Model file for the job. Use its own axes, mm. A direction names the side the tool comes from. Round coordinates to 2 decimals unless told otherwise and drop trailing zeros. Loops run counter-clockwise (first coordinate to the right, second up) from the corner with the lowest first, then second, coordinate; pieces in that order, holes last. Notation, with made-up numbers: (-33.5, 44.25) -> (-15.5, 44.25) arc R14 cw to (-15.5, 63.25) -> close; hole circle Ø3 at (10.25, 50). An arc over 180 degrees is marked (long way). Use a Markdown table: item, result. Add a question column.
```python
from build123d import *

# Parameters (mm, degrees)
F3_DEPTH = 9
F5_DEPTH = 47


with BuildPart() as f1:
    # F0 (on Front) → F1 (revolve)
    with BuildSketch(Plane.XZ):
        Polygon((-5.6564239193, 9.5), (-5.6564239193, 7.5), (19.3435760807, 7.5), (19.3435760807, 9.5), (31.3435760807, 9.5), (31.3435760807, 11.5), (-15.6564239193, 11.5), (-15.6564239193, 9.5), align=None)
    revolve(axis=Axis((2.8128489057, 0, 0), (1, 0, 0)))

    # F2 (on face) → F3 (join)
    with BuildSketch(Plane.YZ.offset(19.3435760807)):
        with BuildLine():
            Line((0, 7.5), (0, 9.5))
            ThreePointArc((0, 9.5), (-1.2098512295, 9.4226461253), (-2.4, 9.191844211))
            Line((-2.4, 9.191844211), (-2.4, 7.5))
            Line((-2.4, 7.5), (0, 7.5))
        make_face()
        with BuildLine():
            ThreePointArc((2.4, 9.191844211), (1.2098512295, 9.4226461253), (0, 9.5))
            Line((0, 9.5), (0, 7.5))
            Line((0, 7.5), (2.4, 7.5))
            Line((2.4, 7.5), (2.4, 9.191844211))
        make_face()
    extrude(amount=F3_DEPTH)

    # F4 (on face) → F5 (join, through all)
    with BuildSketch(Plane.YZ.offset(31.3435760807)):
        with BuildLine():
            Line((-15, -11.5), (0, -11.5))
            ThreePointArc((0, -11.5), (-4.1533119315, -10.7238052948), (-7.7459666924, -8.5))
            Line((-7.7459666924, -8.5), (-15, -8.5))
            Line((-15, -8.5), (-15, -11.5))
        make_face()
        with BuildLine():
            ThreePointArc((7.7459666924, -8.5), (4.1533119315, -10.7238052948), (0, -11.5))
            Line((0, -11.5), (15, -11.5))
            Line((15, -11.5), (15, -8.5))
            Line((15, -8.5), (7.7459666924, -8.5))
        make_face()
    extrude(amount=-F5_DEPTH)


solid = f1.part
```
1) Tool access for faces 4 (the face through (8, 11, -8.5)), 5 (the face through (-5.656, -8, 1)), 6 (the face through (8, -11, -8.5)), 7 (the face through (24, 0, 7.5)): list every direction of +Z, -Z, +X, -X, +Y, -Y with a clear straight run to the whole face (end or side of a thin tool).
2) Cut at D-D on x = 24. Write the cut outline in (y, z), and give its area (3 significant figures).
3) Cut at B-B on x = 7.5. Write the cut outline in (y, z), and give its area (3 significant figures).
4) Cut at C-C on y = -5. Write the cut outline in (x, z).
5) Pull direction Y, two halves, no side cores. Call faces 1 (the face through (28.344, 0, 9)), 2 (the face through (8, -15, -10)), 3 (the face through (-15.656, 0, -10)): +Y half, -Y half, draft (parallel to the pull), parting line (faces both ways), or undercut.
6) Wall check: probe 1 along Y at (x, z) = (-13, 0); probe 2 along Y at (x, z) = (3, 0); probe 3 along Z at (x, y) = (26.25, 0). Give the ranges that are in metal, low to high. Write a range as from..to.
7) Pin check, flat tips, straight feed: pin 1 Ø6 at (x, y) = (6, 10.5) entering from +Z; pin 2 Ø3.5 at (x, y) = (13, -10.5) entering from +Z; pin 3 Ø12 at (x, z) = (0.5, -4) entering from +Y; pin 4 Ø1.5 at (x, z) = (25.5, 0) entering from -Y. Stop position of each tip, or through.
8) Cut at A-A on z = 0. Write the cut outline in (x, y), and give its area (3 significant figures).
Established:
| question | item | result |
|---|---|---|
| 1 | face 4 | +X, -X, +Y |
| 1 | face 5 | -X |
| 1 | face 6 | +X, -X, -Y |
| 1 | face 7 | +X |
| 2 | outline | (-15, -11.5) -> (15, -11.5) -> (15, -8.5) -> (7.75, -8.5) arc R11.5 ccw (long way) to (-7.75, -8.5) -> (-15, -8.5) -> close; hole (-2.4, 7.5) -> (-2.4, 9.19) arc R9.5 ccw (long way) to (2.4, 9.19) -> (2.4, 7.5) -> close |
| 2 | area | 199 mm^2 |
| 3 | outline | (-15, -11.5) -> (15, -11.5) -> (15, -8.5) -> (7.75, -8.5) arc R11.5 ccw (long way) to (-7.75, -8.5) -> (-15, -8.5) -> close; hole circle Ø15 at (0, 0) |
| 3 | area | 297 mm^2 |
| 4 | outline | (-15.66, -11.5) -> (31.34, -11.5) -> (31.34, -8.08) -> (19.34, -8.08) -> (19.34, -5.59) -> (-5.66, -5.59) -> (-5.66, -8.08) -> (-15.66, -8.08) -> close; (-15.66, 8.08) -> (-5.66, 8.08) -> (-5.66, 5.59) -> (19.34, 5.59) -> (19.34, 8.08) -> (31.34, 8.08) -> (31.34, 10.36) -> (-15.66, 10.36) -> close |
| 5 | face 1 | undercut |
| 5 | face 2 | -Y half |
| 5 | face 3 | draft |
| 6 | probe 1 | y = -11.5..-9.5, 9.5..11.5 |
| 6 | probe 2 | y = -11.5..-7.5, 7.5..11.5 |
| 6 | probe 3 | z = -11.5..-9.5, 7.5..11.5 |
| 7 | pin 1 | stops at z = 8.72 |
| 7 | pin 2 | stops at z = 7.46 |
| 7 | pin 3 | stops at y = 15 |
| 7 | pin 4 | stops at y = -11.5 |
| 8 | outline | (-15.66, -11.5) -> (31.34, -11.5) -> (31.34, -9.5) -> (19.34, -9.5) -> (19.34, -7.5) -> (-5.66, -7.5) -> (-5.66, -9.5) -> (-15.66, -9.5) -> close; (-15.66, 9.5) -> (-5.66, 9.5) -> (-5.66, 7.5) -> (19.34, 7.5) -> (19.34, 9.5) -> (31.34, 9.5) -> (31.34, 11.5) -> (-15.66, 11.5) -> close |
| 8 | area | 288 mm^2 |
